Model file for the job. Use its own axes, mm. A direction names the side the tool comes from. Give positions to 0.01 mm unless a question says otherwise; leave off trailing zeros. Write each loop counter-clockwise with the first axis right and the second up, starting at its lowest first coordinate (ties: lowest second). Pieces come first, ordered by that corner, then holes. Notation, with made-up numbers: (78.5, 57) - (135.5, 57) arc R23 ccw to (135.5, 88) - close; hole circle Ø3 at (46, 55). An arc over 180 degrees is marked (long way). One line per item, written item: value. Start each with the question number.
(1) Cut at A-A, the plane y = 116.5. List the corners of the cut face in (x, z), and give its area (3 significant figures).
(2) Probe L1, parallel to Y at x = 50, z = 2.35; L2, parallel to X at y = 207.5, z = 4.45; L3, parallel to Y at x = 54.5, z = 2.3. List the from-to ranges inside material, lowest first.
(3) Cut at B-B, the plane x = 50. List the corners of the cut face in (y, z), and give its area (4 significant figures).
(4) Mould opens along Y. For faces 1 (the face through (50, -35, 3)), 2 (the face through (57.5, -27, 3)), 3 (the face through (49, 0, 3)) say: pulls with the +Y half, pulls with the -Y half, needs draft (parallel to the pull), parting line crosses it, or undercut.
(5) Drop flat-ended pins along their axis: P1, Ø3, axis at x = 107.5, z = 3.5, coming from the +Y side; P2, Ø1.6, axis at x = 85, z = 2, coming from the -Y side; P3, Ø10, axis at x = 3, y = 59, coming from the +Z side. Give the stop position or say it passes through.
(6) Cut at D-D, the plane x = 27. List the corners of the cut face in (y, z).
(7) Cut at C-C, the plane z = 4.55. List the corners of the cut face in (x, y).
(8) 3-axis set-ups, long thin cutter, end or side, ignore diameter. For faces 4 (the face through (42.5, -28, 3)), 5 (the face through (0, 76, 3)), 6 (the face through (88, -20, 3)), 7 (the face through (0, 218, 3)): which of +Z, -Z, +X, -X, +Y, -Y reach the whole face in a straight line?
Autodesk Inventor part; units mm, degrees
ref_plane "YZ Plane" through (0, 0, 0) normal (1, 0, 0) x (0, 1, 0)
ref_plane "XZ Plane" through (0, 0, 0) normal (0, 1, 0) x (-1, 0, 0)
ref_plane "XY Plane" through (0, 0, 0) normal (0, 0, 1) x (1, 0, 0)
sketch "Sketch1" plane through (0, 0, 0) normal (0, 0, 1) x (1, 0, 0)
  line L0 (0, 0) -> (100, 0)
  line L1 (100, 0) -> (100, 150)
  line L2 (100, 150) -> (0, 150)
  line L3 (0, 150) -> (0, 0)
  circle A0 centre (50, 207.5) radius 37.5
  line L4 (-20, -20) -> (120, -20)
  line L5 (120, -20) -> (120, 170)
  line L6 (120, 170) -> (-20, 170)
  line L7 (-20, 170) -> (-20, -20)
  line L8 (0, 170) -> (100, 170)
  line L9 (100, 170) -> (100, 265)
  line L10 (100, 265) -> (0, 265)
  line L11 (0, 265) -> (0, 170)
  line L12 (49.5, -20) -> (59.5, -20)
  line L13 (45, -20) -> (60, -20)
  line L14 (42.5, -20) -> (57.5, -20)
  line L15 (57.5, -20) -> (57.5, -35)
  line L16 (57.5, -35) -> (42.5, -35)
  line L17 (42.5, -35) -> (42.5, -20)
  dimension "d4" = 75
  dimension "d5" = 140
  dimension "d6" = 95
  dimension "d13" = 15
  dimension "d14" = 15
extrude "Extrusion1" add sketch "Sketch1" along normal blind 5.5
properties part number "anillo"
Answers follow:
1. outline: (-20, 0) - (0, 0) - (0, 5.5) - (-20, 5.5) - close; (100, 0) - (120, 0) - (120, 5.5) - (100, 5.5) - close
1. area: 220 mm²
2. L1: y = -35 to 0, 150 to 170, 245 to 265
2. L2: x = 0 to 12.5, 87.5 to 100
2. L3: y = -35 to 0, 150 to 170.27, 244.73 to 265
3. outline: (-35, 0) - (0, 0) - (0, 5.5) - (-35, 5.5) - close; (150, 0) - (170, 0) - (170, 5.5) - (150, 5.5) - close; (245, 0) - (265, 0) - (265, 5.5) - (245, 5.5) - close
3. area: 412.5 mm²
4. face 1: pulls with the -Y half
4. face 2: needs draft
4. face 3: undercut
5. P1: stops at y = 170
5. P2: stops at y = -20
5. P3: stops at z = 5.5
6. outline: (-20, 0) - (0, 0) - (0, 5.5) - (-20, 5.5) - close; (150, 0) - (177.88, 0) - (177.88, 5.5) - (150, 5.5) - close; (237.12, 0) - (265, 0) - (265, 5.5) - (237.12, 5.5) - close
7. outline: (-20, -20) - (42.5, -20) - (42.5, -35) - (57.5, -35) - (57.5, -20) - (120, -20) - (120, 170) - (100, 170) - (100, 265) - (0, 265) - (0, 170) - (-20, 170) - close; hole (0, 0) - (100, 0) - (100, 150) - (0, 150) - close; hole circle Ø75 at (50, 207.5)
8. face 4: +Z, -Z, -X, -Y
8. face 5: +Z, -Z
8. face 6: +Z, -Z, +X, -Y
8. face 7: +Z, -Z, -X, +Y
